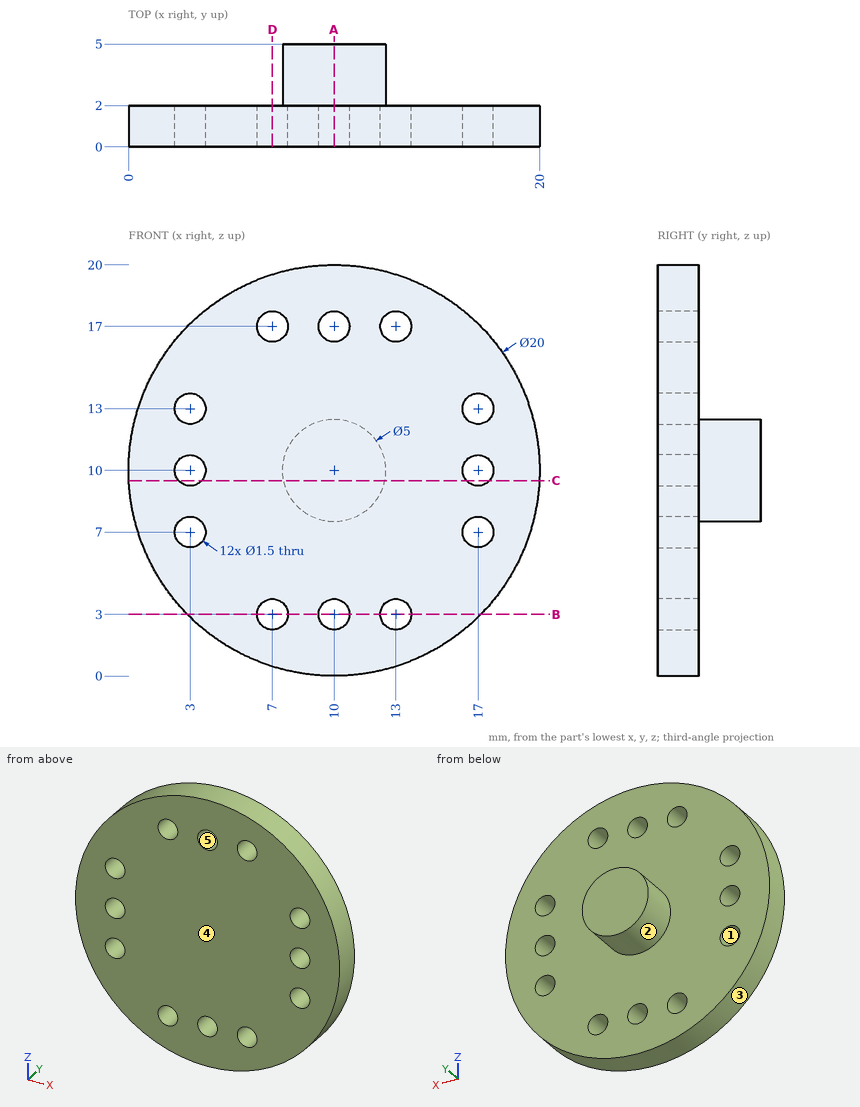
Study the drawing (mm; zero at the part's minimum x, y, z) and answer. A direction names the side the tool comes from. Give positions to 0.01 mm unless a question says otherwise; leave off trailing zeros. Order: outer loops, then holes, each group sorted by start corner. A loop starts at its lowest first (then second) coordinate and runs counter-clockwise, first axis right, second up. Notation, with made-up numbers: (-28.5, -15.5) - (2.5, -15.5) arc R15 cw to (2.5, 9.5) - close; hole circle Ø8 at (79, 11). An arc over 180 degrees is marked (long way). Answer in a Markdown table with one row per item. Add a question column.
Q1. The part is cut by section B-B (z = 3). Determine the outline of the cut face in (x, y), then the cut area to 3 significant figures.
Q2. The part is cut by section D-D (x = 7). Determine the outline of the cut face in (y, z), then the cut area to 3 significant figures.
Q3. Which of the six approach directions +Z, -Z, +X, -X, +Y, -Y give full straight-line access (tool end or side, diameter ignored) to the marked faces 1 and 2?
Q4. The part is cut by section C-C (z = 9.5). Determine the outline of the cut face in (x, y), then the cut area to 3 significant figures.
Q5. For a pull along Z with two mould halves and no side action, classify the marked faces 3, 4 and 5 as released by +Z, released by -Z, zero draft, split by the parting line, or undercut.
Q6. Find the intervals of material crossed by line 1 along X through (y, z) = (0.75, 10); line 2 along X through (y, z) = (0.9, 17); line 3 along Z through (x, y) = (17.25, 1), in increasing order. Write a range as [from, to].
Q7. The part is cut by section A-A (x = 10). Determine the outline of the cut face in (y, z).
Q8. Given P1, Ø3, axis at y = 1, z = 16.5, coming from the -X side; P2, Ø3, axis at x = 7, y = 2.5, coming from the +Z side; P3, Ø1.5, axis at x = 13.5, z = 13.5, coming from the +Y side, each flat-ended and moving along its own axis, determine where each tip first touches the part or whether it passes through.
Determined:
| question | item | result |
|---|---|---|
| 1 | outline | (2.86, 0) - (6.25, 0) - (6.25, 2) - (2.86, 2) - close; (7.75, 0) - (9.25, 0) - (9.25, 2) - (7.75, 2) - close; (10.75, 0) - (12.25, 0) - (12.25, 2) - (10.75, 2) - close; (13.75, 0) - (17.14, 0) - (17.14, 2) - (13.75, 2) - close |
| 1 | area | 19.6 mm² |
| 2 | outline | (0, 0.46) - (2, 0.46) - (2, 2.25) - (0, 2.25) - close; (0, 3.75) - (2, 3.75) - (2, 16.25) - (0, 16.25) - close; (0, 17.75) - (2, 17.75) - (2, 19.54) - (0, 19.54) - close |
| 2 | area | 32.2 mm² |
| 3 | face 1 | +Y, -Y |
| 3 | face 2 | +Y |
| 4 | outline | (0.01, 0) - (2.44, 0) - (2.44, 2) - (0.01, 2) - close; (3.56, 0) - (16.44, 0) - (16.44, 2) - (12.45, 2) - (12.45, 5) - (7.55, 5) - (7.55, 2) - (3.56, 2) - close; (17.56, 0) - (19.99, 0) - (19.99, 2) - (17.56, 2) - close |
| 4 | area | 50.2 mm² |
| 5 | face 3 | split by the parting line |
| 5 | face 4 | zero draft |
| 5 | face 5 | undercut |
| 6 | line 1 | x = [0, 2.25], [3.75, 16.25], [17.75, 20] |
| 6 | line 2 | x = [2.86, 6.25], [7.75, 9.25], [10.75, 12.25], [13.75, 17.14] |
| 6 | line 3 | z = [3.11, 6.29], [7.71, 9.29], [10.71, 12.29], [13.71, 16.89] |
| 7 | outline | (0, 0) - (2, 0) - (2, 2.25) - (0, 2.25) - close; (0, 3.75) - (2, 3.75) - (2, 7.5) - (5, 7.5) - (5, 12.5) - (2, 12.5) - (2, 16.25) - (0, 16.25) - close; (0, 17.75) - (2, 17.75) - (2, 20) - (0, 20) - close |
| 8 | P1 | stops at x = 1.34 |
| 8 | P2 | stops at z = 19.87 |
| 8 | P3 | stops at y = 2 |
